The listing builds one solid part. Answer for the finished solid, in the listing's coordinates (mm). Coordinates: 2 decimals unless noted, no trailing zeros. Write each loop counter-clockwise with the first axis right and the second up, starting at its lowest first coordinate (ties: lowest second). Pieces come first, ordered by that corner, then holes.
from build123d import *

# Parameters (mm, degrees)
F0_W     = 1385.8875
F0_H     = 712.7875
F0_W_2   = 284.1625
F0_H_2   = 182.5625
F0_W_3   = 627.0625
F0_H_3   = 415.925
F0_H_4   = 131.7625
F1_DEPTH = 19.05


with BuildPart() as f1:
    # F0 (on Front) → F1 (new body)
    with BuildSketch(Plane.XZ):
        Rectangle(F0_W, F0_H)
        with Locations((-500.0625, -201.6125)):
            Rectangle(F0_W_2, F0_H_2, mode=Mode.SUBTRACT)
        with Locations((0, -84.93125)):
            Rectangle(F0_W_3, F0_H_3, mode=Mode.SUBTRACT)
        with Locations((500.0625, -201.6125)):
            Rectangle(F0_W_2, F0_H_2, mode=Mode.SUBTRACT)
        with Locations((-500.0625, 31.75)):
            Rectangle(F0_W_2, F0_H_2, mode=Mode.SUBTRACT)
        with Locations((-500.0625, 239.7125)):
            Rectangle(F0_W_2, F0_H_4, mode=Mode.SUBTRACT)
        with Locations((0, 239.7125)):
            Rectangle(F0_W_3, F0_H_4, mode=Mode.SUBTRACT)
        with Locations((500.0625, 31.75)):
            Rectangle(F0_W_2, F0_H_2, mode=Mode.SUBTRACT)
        with Locations((500.0625, 239.7125)):
            Rectangle(F0_W_2, F0_H_4, mode=Mode.SUBTRACT)
    extrude(amount=F1_DEPTH)


solid = f1.part
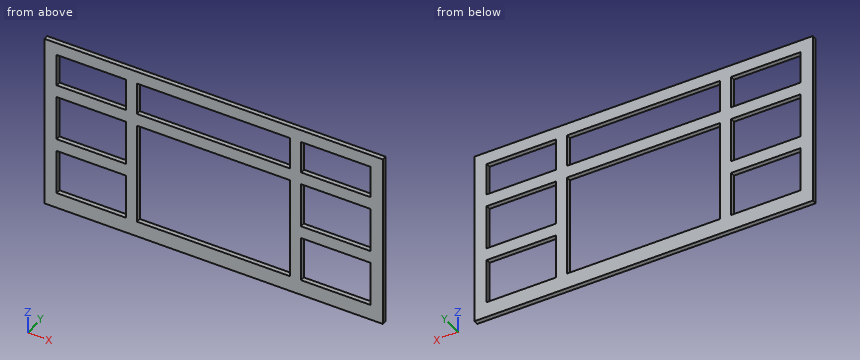
1. Section C-C on x = -501.5 is taken. Give the vertices of the cut face in (y, z), then the cut area to 3 significant figures.
Results found:
outline: (-19.05, -356.39) - (0, -356.39) - (0, -292.89) - (-19.05, -292.89) - close; (-19.05, -110.33) - (0, -110.33) - (0, -59.53) - (-19.05, -59.53) - close; (-19.05, 123.03) - (0, 123.03) - (0, 173.83) - (-19.05, 173.83) - close; (-19.05, 305.59) - (0, 305.59) - (0, 356.39) - (-19.05, 356.39) - close
area: 4,110 mm2
2. Section D-D on y = -7.5 is taken. State how many separate pieces and enclosed holes the cut face has, then the cut area to 3 significant figures.
Results found:
separate pieces: 1
enclosed holes: 8
area: 362,000 mm2
3. Section B-B on z = -229 is taken. Give the vertices of the cut face in (x, y).
Results found:
outline: (-692.94, -19.05) - (-642.14, -19.05) - (-642.14, 0) - (-692.94, 0) - close; (-357.98, -19.05) - (-313.53, -19.05) - (-313.53, 0) - (-357.98, 0) - close; (313.53, -19.05) - (357.98, -19.05) - (357.98, 0) - (313.53, 0) - close; (642.14, -19.05) - (692.94, -19.05) - (692.94, 0) - (642.14, 0) - close
4. Find the intervals of material crossed by L1, parallel to Z at x = 513, y = -2.5; L2, parallel to X at y = -2.5, z = 203; L3, parallel to Z at x = -117.5, y = -3.5, in increasing order.
Results found:
L1: z = -356.39 to -292.89, -110.33 to -59.53, 123.03 to 173.83, 305.59 to 356.39
L2: x = -692.94 to -642.14, -357.98 to -313.53, 313.53 to 357.98, 642.14 to 692.94
L3: z = -356.39 to -292.89, 123.03 to 173.83, 305.59 to 356.39
5. Section A-A on x = 238 is taken. Give the vertices of the cut face in (y, z), then the cut area to 3 significant figures.
Results found:
outline: (-19.05, -356.39) - (0, -356.39) - (0, -292.89) - (-19.05, -292.89) - close; (-19.05, 123.03) - (0, 123.03) - (0, 173.83) - (-19.05, 173.83) - close; (-19.05, 305.59) - (0, 305.59) - (0, 356.39) - (-19.05, 356.39) - close
area: 3,150 mm2
